```python
from build123d import *

# Parameters (mm, degrees)
SKETCH1_R           = 2
SKETCH1_R_2         = 3
BOSS_EXTRUDE1_DEPTH = 2
CUT_EXTRUDE1_DEPTH  = 3
SKETCH3_W           = 158.631483428
SKETCH3_H           = 58.126698801
CUT_EXTRUDE2_DEPTH  = 3


with BuildPart() as part:
    # Sketch1 → Boss-Extrude1 (new body)
    with BuildSketch(Plane.XY):
        with BuildLine():
            Line((236, -43.5), (-236, -43.5))
            Line((-236, -43.5), (-239.5, -43.5))
            ThreePointArc((-239.5, -43.5), (-240.560660172, -43.060660172), (-241, -42))
            Line((-241, -42), (-241, -38.5))
            Line((-241, -38.5), (-241, 38.5))
            Line((-241, 38.5), (-241, 42))
            ThreePointArc((-241, 42), (-240.560660172, 43.060660172), (-239.5, 43.5))
            Line((-239.5, 43.5), (-236, 43.5))
            Line((-236, 43.5), (236, 43.5))
            Line((236, 43.5), (239.5, 43.5))
            ThreePointArc((239.5, 43.5), (240.560660172, 43.060660172), (241, 42))
            Line((241, 42), (241, 38.5))
            Line((241, 38.5), (241, -38.5))
            Line((241, -38.5), (241, -42))
            ThreePointArc((241, -42), (240.560660172, -43.060660172), (239.5, -43.5))
            Line((239.5, -43.5), (236, -43.5))
        make_face()
        with Locations((-200.85, 30)):
            Circle(SKETCH1_R, mode=Mode.SUBTRACT)
        with Locations((-200.85, 0)):
            Circle(SKETCH1_R, mode=Mode.SUBTRACT)
        with Locations((-200.85, -30)):
            Circle(SKETCH1_R, mode=Mode.SUBTRACT)
        with Locations((200.85, 30)):
            Circle(SKETCH1_R, mode=Mode.SUBTRACT)
        with Locations((200.85, 0)):
            Circle(SKETCH1_R, mode=Mode.SUBTRACT)
        with Locations((200.85, -30)):
            Circle(SKETCH1_R, mode=Mode.SUBTRACT)
        with Locations((0, -27.56)):
            Circle(SKETCH1_R_2, mode=Mode.SUBTRACT)
        with Locations((0, 27.56)):
            Circle(SKETCH1_R_2, mode=Mode.SUBTRACT)
        with BuildLine():
            Line((-235, 34.6), (-230, 34.6))
            ThreePointArc((-230, 34.6), (-226.5, 38.1), (-230, 41.6))
            Line((-230, 41.6), (-235, 41.6))
            ThreePointArc((-235, 41.6), (-238.5, 38.1), (-235, 34.6))
        make_face(mode=Mode.SUBTRACT)
        with BuildLine():
            Line((-235, -41.6), (-230, -41.6))
            ThreePointArc((-230, -41.6), (-226.5, -38.1), (-230, -34.6))
            Line((-230, -34.6), (-235, -34.6))
            ThreePointArc((-235, -34.6), (-238.5, -38.1), (-235, -41.6))
        make_face(mode=Mode.SUBTRACT)
        with BuildLine():
            Line((235, -41.6), (230, -41.6))
            ThreePointArc((230, -41.6), (226.5, -38.1), (230, -34.6))
            Line((230, -34.6), (235, -34.6))
            ThreePointArc((235, -34.6), (238.5, -38.1), (235, -41.6))
        make_face(mode=Mode.SUBTRACT)
        with BuildLine():
            Line((230, 41.6), (235, 41.6))
            ThreePointArc((235, 41.6), (238.5, 38.1), (235, 34.6))
            Line((235, 34.6), (230, 34.6))
            ThreePointArc((230, 34.6), (226.5, 38.1), (230, 41.6))
        make_face(mode=Mode.SUBTRACT)
    extrude(amount=BOSS_EXTRUDE1_DEPTH)

    # Sketch2 → Cut-Extrude1 (cut)
    with BuildSketch(Plane.XY.offset(2)):
        with BuildLine():
            Line((124.488551372, 16.409445117), (124.488551372, 38.909445117))
            ThreePointArc((124.488551372, 38.909445117), (133.667112168, 37.768818347), (142.28730965, 34.416326275))
            Line((142.28730965, 34.416326275), (131.608054683, 14.61219758))
            ThreePointArc((131.608054683, 14.61219758), (128.159975691, 15.953194409), (124.488551372, 16.409445117))
        make_face()
        with BuildLine():
            Line((138.858556239, 5.710951844), (160.41356354, 12.163211934))
            ThreePointArc((160.41356354, 12.163211934), (156.688733324, 20.629181907), (151.005055666, 27.925949412))
            Line((151.005055666, 27.925949412), (135.09515309, 12.016046835))
            ThreePointArc((135.09515309, 12.016046835), (137.368624153, 9.097339833), (138.858556239, 5.710951844))
        make_face()
        with BuildLine():
            Line((137.691303835, -5.710058194), (157.49543253, -16.389313161))
            ThreePointArc((157.49543253, -16.389313161), (160.847924602, -7.769115679), (161.988551372, 1.409445117))
            Line((161.988551372, 1.409445117), (139.488551372, 1.409445117))
            ThreePointArc((139.488551372, 1.409445117), (139.032300664, -2.261979201), (137.691303835, -5.710058194))
        make_face()
        with BuildLine():
            Line((128.790058099, -12.96055975), (135.242318189, -34.51556705))
            ThreePointArc((135.242318189, -34.51556705), (143.708288162, -30.790736834), (151.005055666, -25.107059177))
            Line((151.005055666, -25.107059177), (135.09515309, -9.197156601))
            ThreePointArc((135.09515309, -9.197156601), (132.176446088, -11.470627664), (128.790058099, -12.96055975))
        make_face()
        with BuildLine():
            Line((117.369048061, -11.793307346), (106.689793094, -31.59743604))
            ThreePointArc((106.689793094, -31.59743604), (115.309990575, -34.949928113), (124.488551372, -36.090554883))
            Line((124.488551372, -36.090554883), (124.488551372, -13.590554883))
            ThreePointArc((124.488551372, -13.590554883), (120.817127053, -13.134304175), (117.369048061, -11.793307346))
        make_face()
        with BuildLine():
            Line((110.118546505, -2.89206161), (88.563539204, -9.3443217))
            ThreePointArc((88.563539204, -9.3443217), (92.28836942, -17.810291673), (97.972047077, -25.107059177))
            Line((97.972047077, -25.107059177), (113.881949654, -9.197156601))
            ThreePointArc((113.881949654, -9.197156601), (111.608478591, -6.278449599), (110.118546505, -2.89206161))
        make_face()
        with BuildLine():
            Line((111.285798909, 8.528948428), (91.481670214, 19.208203395))
            ThreePointArc((91.481670214, 19.208203395), (88.129178142, 10.588005914), (86.988551372, 1.409445117))
            Line((86.988551372, 1.409445117), (109.488551372, 1.409445117))
            ThreePointArc((109.488551372, 1.409445117), (109.94480208, 5.080869436), (111.285798909, 8.528948428))
        make_face()
        with BuildLine():
            Line((120.187044645, 15.779449984), (113.734784555, 37.334457285))
            ThreePointArc((113.734784555, 37.334457285), (105.268814582, 33.609627069), (97.972047077, 27.925949412))
            Line((97.972047077, 27.925949412), (113.881949654, 12.016046835))
            ThreePointArc((113.881949654, 12.016046835), (116.800656656, 14.289517898), (120.187044645, 15.779449984))
        make_face()
        with BuildLine():
            Line((53.433328256, 12.016046835), (69.343230833, 27.925949412))
            ThreePointArc((69.343230833, 27.925949412), (62.046463328, 33.609627069), (53.580493355, 37.334457285))
            Line((53.580493355, 37.334457285), (47.128233265, 15.779449984))
            ThreePointArc((47.128233265, 15.779449984), (50.514621254, 14.289517898), (53.433328256, 12.016046835))
        make_face()
        with BuildLine():
            Line((57.826726538, 1.409445117), (80.326726538, 1.409445117))
            ThreePointArc((80.326726538, 1.409445117), (79.186099769, 10.588005914), (75.833607696, 19.208203395))
            Line((75.833607696, 19.208203395), (56.029479001, 8.528948428))
            ThreePointArc((56.029479001, 8.528948428), (57.37047583, 5.080869436), (57.826726538, 1.409445117))
        make_face()
        with BuildLine():
            Line((53.433328256, -9.197156601), (69.343230833, -25.107059177))
            ThreePointArc((69.343230833, -25.107059177), (75.02690849, -17.810291673), (78.751738706, -9.3443217))
            Line((78.751738706, -9.3443217), (57.196731405, -2.89206161))
            ThreePointArc((57.196731405, -2.89206161), (55.706799319, -6.278449599), (53.433328256, -9.197156601))
        make_face()
        with BuildLine():
            Line((42.826726538, -13.590554883), (42.826726538, -36.090554883))
            ThreePointArc((42.826726538, -36.090554883), (52.005287335, -34.949928113), (60.625484817, -31.59743604))
            Line((60.625484817, -31.59743604), (49.94622985, -11.793307346))
            ThreePointArc((49.94622985, -11.793307346), (46.498150857, -13.134304175), (42.826726538, -13.590554883))
        make_face()
        with BuildLine():
            Line((32.22012482, -9.197156601), (16.310222244, -25.107059177))
            ThreePointArc((16.310222244, -25.107059177), (23.606989748, -30.790736834), (32.072959721, -34.51556705))
            Line((32.072959721, -34.51556705), (38.525219811, -12.96055975))
            ThreePointArc((38.525219811, -12.96055975), (35.138831822, -11.470627664), (32.22012482, -9.197156601))
        make_face()
        with BuildLine():
            Line((27.826726538, 1.409445117), (5.326726538, 1.409445117))
            ThreePointArc((5.326726538, 1.409445117), (6.467353308, -7.769115679), (9.819845381, -16.389313161))
            Line((9.819845381, -16.389313161), (29.623974075, -5.710058194))
            ThreePointArc((29.623974075, -5.710058194), (28.282977246, -2.261979201), (27.826726538, 1.409445117))
        make_face()
        with BuildLine():
            Line((32.22012482, 12.016046835), (16.310222244, 27.925949412))
            ThreePointArc((16.310222244, 27.925949412), (10.626544587, 20.629181907), (6.901714371, 12.163211934))
            Line((6.901714371, 12.163211934), (28.456721671, 5.710951844))
            ThreePointArc((28.456721671, 5.710951844), (29.946653758, 9.097339833), (32.22012482, 12.016046835))
        make_face()
        with BuildLine():
            Line((35.707223227, 14.61219758), (25.02796826, 34.416326275))
            ThreePointArc((25.02796826, 34.416326275), (33.648165742, 37.768818347), (42.826726538, 38.909445117))
            Line((42.826726538, 38.909445117), (42.826726538, 16.409445117))
            ThreePointArc((42.826726538, 16.409445117), (39.15530222, 15.953194409), (35.707223227, 14.61219758))
        make_face()
    extrude(amount=-CUT_EXTRUDE1_DEPTH, mode=Mode.SUBTRACT)

    # Sketch3 → Cut-Extrude2 (cut)
    with BuildSketch(Plane.XY.offset(2)):
        with Locations((-101.172577856, -1.541774354)):
            Rectangle(SKETCH3_W, SKETCH3_H)
    extrude(amount=-CUT_EXTRUDE2_DEPTH, mode=Mode.SUBTRACT)


solid = part.part
```
CAD build for the part. Positions are in the model's coordinates, mm. A direction names the side the tool comes from. Give positions to 0.01 mm unless a question says otherwise; leave off trailing zeros. Use a Markdown table: item, result.
1. Wall check: L1, parallel to Y at x = 200.85, z = 0.45; L2, parallel to Y at x = -148, z = 1.05; L3, parallel to X at y = -37, z = 1.5. Give the ranges that are in metal, low to high. Write a range as [from, to].
Check result:
| item | result |
|---|---|
| L1 | y = [-43.5, -32], [-28, -2], [2, 28], [32, 43.5] |
| L2 | y = [-43.5, -30.61], [27.52, 43.5] |
| L3 | x = [-241, -238.32], [-226.68, 226.68], [238.32, 241] |
2. Flat gauge pin, fed straight in: pin 1 (3 mm diameter, centred on x = -200.85, y = -30, fed in from -Z) (1 decimal). Where does the tip first touch, or does it go through?
Check result:
| item | result |
|---|---|
| pin 1 | passes through |
3. Mould opens along X. For faces 1 (the cylindrical face through (74.96, -17.92, 1.01)), 2 (the flat face through (3, 1, 0)) say: pulls with the +X half, pulls with the -X half, needs draft (parallel to the pull), parting line crosses it, or undercut.
Check result:
| item | result |
|---|---|
| face 1 | undercut |
| face 2 | needs draft |
4. Slice it at A-A (z = 0.7). Give the number of separate pieces and of enclosed holes in the cut face, plus the area to 3 significant figures.
Check result:
| item | result |
|---|---|
| separate pieces | 1 |
| enclosed holes | 29 |
| area | 27,600 mm^2 |
5. Which spindle directions (+Z, -Z, +X, -X, +Y, -Y) get a long thin tool onto all of the face, cutting with end or side? Do faces 3 (the flat face through (3, 1, 2)), 4 (the cylindrical face through (156.755, 20.518, 1.014)). Say none if no direction does.
Check result:
| item | result |
|---|---|
| face 3 | +Z, +X, -X, +Y, -Y |
| face 4 | +Z, -Z |
